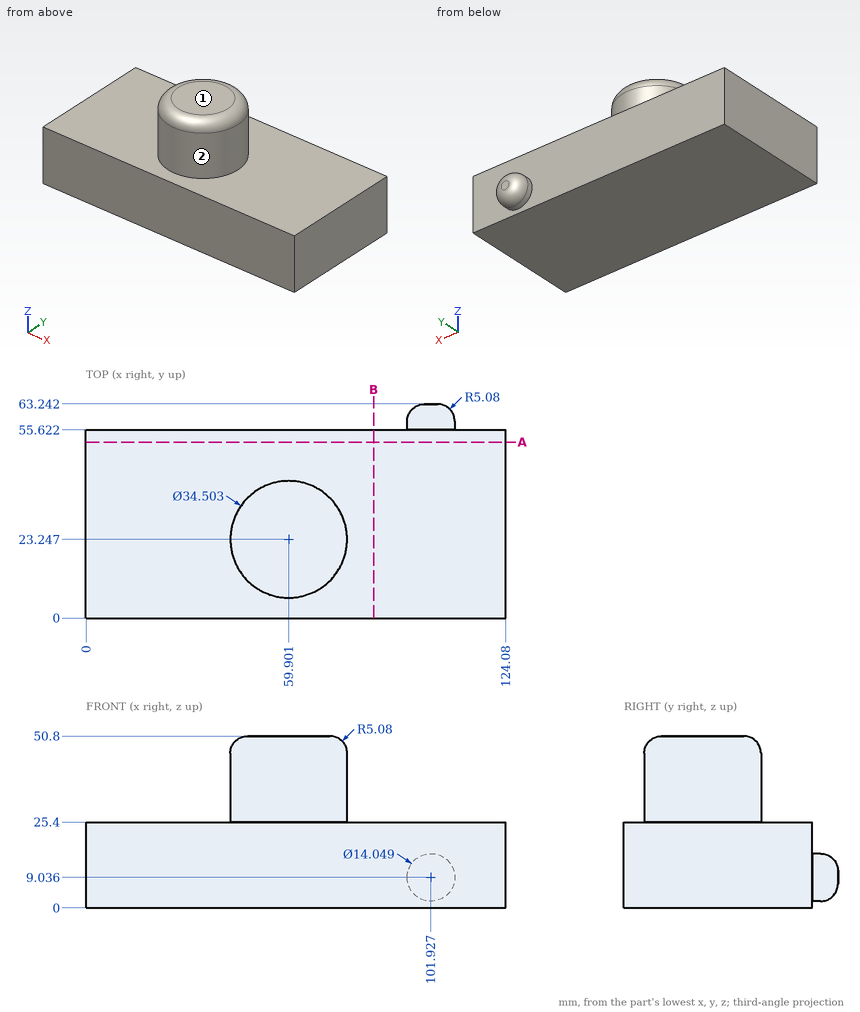
Verification items for this drawing (mm, ordinates from the low corner). A direction names the side the tool comes from. Round coordinates to 2 decimals unless told otherwise and drop trailing zeros. Order: outer loops, then holes, each group sorted by start corner. A loop starts at its lowest first (then second) coordinate and runs counter-clockwise, first axis right, second up. Notation, with made-up numbers: M -33.75,-34 L 14.25,-34 A22 cw 14.25,-16 Z; hole C -31.75,-34.75 d5. An arc over 180 degrees is marked long. Answer in a Markdown table with one row per item. Add a question column.
Item 1: Sectioned sample at B-B, the plane x = 85. Enter the section's corners in (y, z), plus the area to 3 significant figures.
Item 2: Sectioned sample at A-A, the plane y = 52. Enter the section's corners in (x, z).
Item 3: Depth check by flat-ended pin: pin 1 Ø12.5 at (x, z) = (52.5, 10) entering from +Y; pin 2 Ø4 at (x, y) = (18, 25.5) entering from +Z; pin 3 Ø3 at (x, z) = (75.5, 34) entering from -Y (1 decimal). Enter the tip coordinate at first touch or a pass-through.
Item 4: Set-up check for the marked faces 1 and 2: record each of +Z, -Z, +X, -X, +Y, -Y from which the full face is reachable in a straight line by a thin tool's end or side.
Item 5: Material ranges on L1, parallel to Z at x = 72, y = 9; L2, parallel to Y at x = 19.5, z = 8; L3, parallel to Y at x = 57.5, z = 30, recorded low to high. Write a range as [from, to].
Filled in:
| question | item | result |
|---|---|---|
| 1 | outline | M 0,0 L 55.62,0 L 55.62,25.4 L 0,25.4 Z |
| 1 | area | 1,410 mm² |
| 2 | outline | M 0,0 L 124.08,0 L 124.08,25.4 L 0,25.4 Z |
| 3 | pin 1 | stops at y = 55.62 |
| 3 | pin 2 | stops at z = 25.4 |
| 3 | pin 3 | stops at y = 13.3 |
| 4 | face 1 | +Z, +X, -X, +Y, -Y |
| 4 | face 2 | +Z |
| 5 | L1 | z = [0, 25.4] |
| 5 | L2 | y = [0, 55.62] |
| 5 | L3 | y = [6.16, 40.33] |
